For this review, use the dimensioned drawing (mm, ordinates from the lowest corner) and the shaded views. Round coordinates to 2 decimals unless told otherwise and drop trailing zeros. Loops run counter-clockwise (first coordinate to the right, second up) from the corner with the lowest first, then second, coordinate; pieces in that order, holes last.
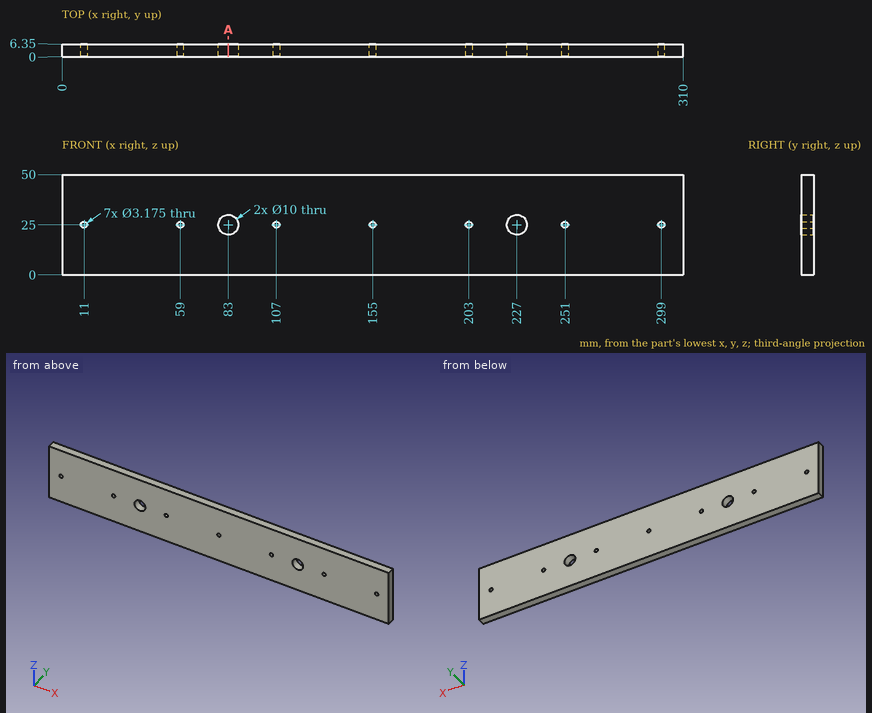
(1) For L1, parallel to Z at x = 299, y = 2.5; L2, parallel to X at y = 2.25, z = 27; L3, parallel to Z at x = 83, y = 3.5, list the stretches that pass through material, from the lowest coordinate up.
(2) Insertion check: pin 1 Ø3 at (x, z) = (203, 25) entering from +Y. The pin has a flat end and moves straight along its axis. Give the tip position at first contact, or say it passes through.
(3) Add section A-A (x = 83). Give the boundary of the cut face in (y, z).
Outcome:
1. L1: z = 0 to 23.41, 26.59 to 50
1. L2: x = 0 to 78.42, 87.58 to 222.42, 231.58 to 310
1. L3: z = 0 to 20, 30 to 50
2. pin 1: passes through
3. outline: (0, 0) - (6.35, 0) - (6.35, 20) - (0, 20) - close; (0, 30) - (6.35, 30) - (6.35, 50) - (0, 50) - close
